Check sheet for the modelled part. Datum: model origin and axes. Units: mm. A direction names the side the tool comes from. Give positions to 0.01 mm unless a question says otherwise; leave off trailing zeros. Order: outer loops, then holes, each group sorted by start corner. A loop starts at its lowest first (then second) coordinate and runs counter-clockwise, first axis right, second up.
```python
from build123d import *

# Parameters (mm, degrees)
F0_W     = 19.36434
F0_H     = 19.05
F1_DEPTH = 57.15
F2_W     = 19.36434
F2_H     = 19.065039
F3_DEPTH = 19.05
F4_W     = 19.05
F4_H     = 18.74761
F5_DEPTH = 19.05


with BuildPart() as f1:
    # F0 (on Top) → F1 (new body)
    with BuildSketch(Plane.XY):
        with Locations((-28.756759, -28.575)):
            Rectangle(F0_W, F0_H)
    extrude(amount=F1_DEPTH)

    # F2 (on face) → F3 (join)
    with BuildSketch(Plane.XZ.offset(38.1)):
        with Locations((-28.756759, 28.86987)):
            Rectangle(F2_W, F2_H)
    extrude(amount=F3_DEPTH)

    # F4 (on face) → F5 (join)
    with BuildSketch(Plane.YZ.offset(-19.074589)):
        with Locations((-28.575, 47.776195)):
            Rectangle(F4_W, F4_H)
    extrude(amount=F5_DEPTH)


solid = f1.part
```
(1) Sectioned sample at D-D (y = -46). Enter the section's corners in (x, z).
(2) Thickness scan on L1, parallel to X at y = -22.5, z = 18; L2, parallel to Z at x = -25, y = -41; L3, parallel to Z at x = -15, y = -34. Record the ranges inside material, lowest first.
(3) Sectioned sample at C-C (z = 15). Enter the section's corners in (x, y).
(4) Go/stop test with flat-tipped pins: P1, Ø19, axis at y = -37.5, z = 25, coming from the +X side; P2, Ø15, axis at x = -23.5, z = 47, coming from the -Y side; P3, Ø15, axis at x = -33, y = -48, coming from the -Z side. Record where each tip stops, or that it passes through.
(5) Tool access check on faces 1 (the face through (-10, -29, 38.402)), 2 (the face through (-29, -47, 38.402)), 3 (the face through (-29, -47, 19.337)). Record the directions out of +Z, -Z, +X, -X, +Y, -Y that give a thin tool (end or side, any length) a straight path to the whole face; none if there is none.
(6) Sectioned sample at A-A (x = -20). Enter the section's corners in (y, z), plus the area to 3 significant figures.
(7) Sectioned sample at B-B (y = -20.5). Enter the section's corners in (x, z), plus the area to 3 significant figures.
Values follow:
1. outline: (-38.44, 19.34) - (-19.07, 19.34) - (-19.07, 38.4) - (-38.44, 38.4) - close
2. L1: x = -38.44 to -19.07
2. L2: z = 19.34 to 38.4
2. L3: z = 38.4 to 57.15
3. outline: (-38.44, -38.1) - (-19.07, -38.1) - (-19.07, -19.05) - (-38.44, -19.05) - close
4. P1: stops at x = -19.07
4. P2: stops at y = -38.1
4. P3: stops at z = 19.34
5. face 1: -Z, +X, +Y, -Y
5. face 2: +Z, +X, -X, -Y
5. face 3: -Z, +X, -X, -Y
6. outline: (-57.15, 19.34) - (-38.1, 19.34) - (-38.1, 0) - (-19.05, 0) - (-19.05, 57.15) - (-38.1, 57.15) - (-38.1, 38.4) - (-57.15, 38.4) - close
6. area: 1,450 mm2
7. outline: (-38.44, 0) - (-19.07, 0) - (-19.07, 38.4) - (-0.02, 38.4) - (-0.02, 57.15) - (-38.44, 57.15) - close
7. area: 1,460 mm2
